The model under review builds one solid part; all positions refer to its coordinate system, in mm. A direction names the side the tool comes from. Give positions to 0.01 mm unless a question says otherwise; leave off trailing zeros. Loops run counter-clockwise (first coordinate to the right, second up) from the corner with the lowest first, then second, coordinate; pieces in that order, holes last. Notation, with made-up numbers: (16, -18.5) - (44, -18.5) arc R21 ccw to (44, -7.5) - close; hole circle Ø3 at (-35.75, -7). An arc over 180 degrees is marked (long way). Answer as a JSON object with one key per item and string values.
from build123d import *

# Parameters (mm, degrees)
F0_W     = 102
F0_H     = 40
F1_DEPTH = 3
F2_W     = 3
F2_H     = 5
F3_DEPTH = 3
F4_W     = 5
F4_H     = 3
F5_DEPTH = 3
F6_W     = 108
F6_H     = 20
F7_DEPTH = 25


with BuildPart() as f1:
    # F0 (on Front) → F1 (new body)
    with BuildSketch(Plane.XZ):
        Rectangle(F0_W, F0_H)
    extrude(amount=F1_DEPTH)

    # F2 (on face) → F3 (join)
    with BuildSketch(Plane.XZ.offset(3)):
        with Locations((-52.5, -17.5)):
            Rectangle(F2_W, F2_H)
        with Locations((-52.5, -7.5)):
            Rectangle(F2_W, F2_H)
        with Locations((-52.5, 2.5)):
            Rectangle(F2_W, F2_H)
        with Locations((-52.5, 12.5)):
            Rectangle(F2_W, F2_H)
        with Locations((52.5, -7.5)):
            Rectangle(F2_W, F2_H)
        with Locations((52.5, -17.5)):
            Rectangle(F2_W, F2_H)
        with Locations((52.5, 12.5)):
            Rectangle(F2_W, F2_H)
        with Locations((52.5, 2.5)):
            Rectangle(F2_W, F2_H)
    extrude(amount=-F3_DEPTH)

    # F4 (on face) → F5 (join)
    with BuildSketch(Plane(origin=(0, 0, 0), x_dir=(-1, 0, 0), z_dir=(0, 1, 0))):
        with Locations((0, 21.5)):
            Rectangle(F4_W, F4_H)
        with Locations((10, 21.5)):
            Rectangle(F4_W, F4_H)
        with Locations((20, 21.5)):
            Rectangle(F4_W, F4_H)
        with Locations((30, 21.5)):
            Rectangle(F4_W, F4_H)
        with Locations((40, 21.5)):
            Rectangle(F4_W, F4_H)
        Polygon((52.5, 23), (47.5, 23), (47.5, 20), (52.5, 20), (54, 20), (54, 23), align=None)
        Polygon((-52.5, 20), (-47.5, 20), (-47.5, 23), (-52.5, 23), (-54, 23), (-54, 20), align=None)
        with Locations((-20, 21.5)):
            Rectangle(F4_W, F4_H)
        with Locations((-10, 21.5)):
            Rectangle(F4_W, F4_H)
        with Locations((-30, 21.5)):
            Rectangle(F4_W, F4_H)
        with Locations((-40, 21.5)):
            Rectangle(F4_W, F4_H)
    extrude(amount=-F5_DEPTH)

    # F6 (on face) → F7 (cut)
    with BuildSketch(Plane(origin=(0, 0, 0), x_dir=(-1, 0, 0), z_dir=(0, 1, 0))):
        with Locations((0, -10)):
            Rectangle(F6_W, F6_H)
    extrude(amount=-F7_DEPTH, mode=Mode.SUBTRACT)


solid = f1.part
Q1. To check wall thickness, follow probe 1 along Z at (x, y) = (-44, -1.1); probe 2 along X at (y, z) = (-0.8, 19.75). State the ranges of each line that lie inside material, in increasing order. Write a range as [from, to].
Results:
{"probe 1": "z = [0, 20]", "probe 2": "x = [-51, 51]"}
Q2. Clearance check with flat-ended pins moving along their axes: pin 1 Ø0.9 at (x, y) = (-26, -1) entering from +Z; pin 2 Ø0.9 at (y, z) = (-2, 17) entering from -X. State where each tip first meets the part, or that it passes through.
Results:
{"pin 1": "stops at z = 20", "pin 2": "stops at x = -51"}
Q3. For faces 1 (the face through (20, -1, 23)), 2 (the face through (47.5, -1, 21)), 3 (the face through (-51, -1, 7)), 4 (the face through (51, -1, 17)), list the 3-axis set-ups (+Z, -Z, +X, -X, +Y, -Y) from which the entire face can be reached by the end or side of a thin tool; tool diameter is ignored.
Results:
{"face 1": "+Z, +X, -X, +Y, -Y", "face 2": "+Z, +Y, -Y", "face 3": "-X, +Y, -Y", "face 4": "+X, +Y, -Y"}
Q4. Consider section A-A, the plane z = 18.75. State the section outline as (x, y) points.
Results:
{"outline": "(-51, -3) - (51, -3) - (51, 0) - (-51, 0) - close"}
Q5. Consider section B-B, the plane x = -36.5. State the section outline as (y, z) points.
Results:
{"outline": "(-3, 0) - (0, 0) - (0, 20) - (-3, 20) - close"}
Q6. The part is to be moulded in two halves that separate along Z. For faces 5 (the face through (-52, -1, 20)), 6 (the face through (-12.5, -1, 21)), 7 (the face through (15, -1, 20)), say which applies: +Z half, -Z half, draft (parallel to the pull), parting line (faces both ways), or undercut.
Results:
{"face 5": "undercut", "face 6": "draft", "face 7": "+Z half"}
